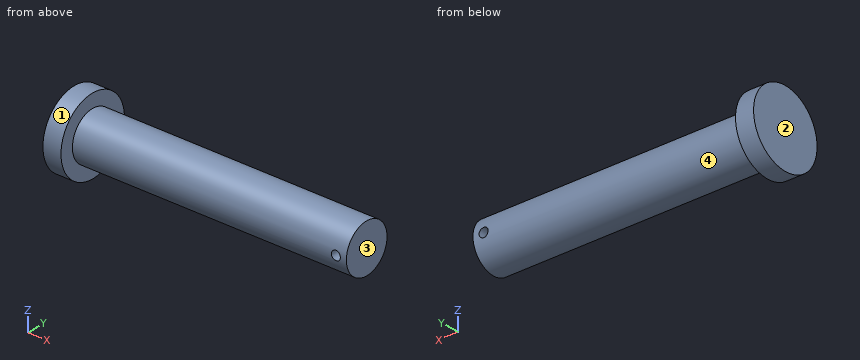
Autodesk Inventor part; units mm, degrees
ref_plane "Work Plane1" through (0, 16, 0) normal (0, 1, 0) x (-1, 0, 0)
ref_plane "YZ Plane" through (0, 0, 0) normal (1, 0, 0) x (0, 1, 0)
ref_plane "XY Plane" through (0, 0, 0) normal (0, 0, 1) x (1, 0, 0)
sketch "Sketch1" plane through (0, 0, 0) normal (1, 0, 0) x (0, 1, 0)
  line L0 (0, 35) -> (0, -35)
  line L1 (-35, 0) -> (35, 0)
  circle A0 centre (0, 0) radius 25
  dimension "d0" = 50
extrude "Extrusion1" add sketch "Sketch1" along normal blind 12
sketch "Sketch2" plane through (12, 0, 0) normal (1, 0, 0) x (0, 0, -1)
  circle A0 centre (0, 0) radius 16
  dimension "d3" = 32
extrude "Extrusion2" add sketch "Sketch2" along normal blind 182
ref_plane "Work Plane1" through (0, 16, 0) normal (0, 1, 0) x (-1, 0, 0)
sketch "Sketch3" plane through (0, 16, 0) normal (0, 1, 0) x (-1, 0, 0)
  circle A0 centre (-187, 0) radius 3
  point P0 (0, 0)
  dimension "d7" = 6
extrude "Extrusion3" cut sketch "Sketch3" against normal through all
properties part number "Pin" material "Stainless Steel"
Input: part model. Units: mm. Frame: model coordinates. Face numbers are marked on the shaded views. A direction names the side the tool comes from. Coordinates: 2 decimals unless noted, no trailing zeros. Order: outer loops, then holes, each group sorted by start corner. A loop starts at its lowest first (then second) coordinate and runs counter-clockwise, first axis right, second up. Notation, with made-up numbers: M 67.5,25.5 L 101.5,25.5 A15 ccw 101.5,31.5 Z; hole C 45.25,43 d11. An arc over 180 degrees is marked long. Write item = value, one per line. Start each with the question number.
(1) Line query: line 1 along X through (y, z) = (8, 0); line 2 along Z through (x, y) = (187, -0.5); line 3 along X through (y, z) = (17, 5). Output: solid intervals per line, ascending. Write a range as [from, to].
(2) First-contact query: P1, Ø1.5, axis at x = 154, z = -3, coming from the -Y side; P2, Ø12, axis at x = 171.5, z = -14.5, coming from the -Y side; P3, Ø10, axis at x = 121.5, z = 0, coming from the -Y side. Flat tips, straight axial feed; report the tip coordinate or a pass-through.
(3) Pull-direction query (Z, two-part tool) for the marked faces 1 and 2; classes: released by +Z, released by -Z, zero draft, split by the parting line, or undercut.
(4) Section C-C on x = 101. Output: boundary loops of the cut face in (y, z).
(5) Section A-A on z = 0. Output: boundary loops of the cut face in (x, y), and give its area (3 significant figures).
(6) Section B-B on y = 0. Output: boundary loops of the cut face in (x, z).
(7) Reachability of the marked faces 3 and 4 from +Z, -Z, +X, -X, +Y, -Y: full face, straight path, thin tool, end or side. Return the list, or none.
(8) Section D-D on z = 8.5. Output: boundary loops of the cut face in (x, y).
Result set:
q1.line_1 = [0, 184], [190, 194]
q1.line_2 = [-15.99, -3], [3, 15.99]
q1.line_3 = [0, 12]
q2.P1 = -15.84
q2.P2 = -13.56
q2.P3 = -16
q3.face_1 = split by the parting line
q3.face_2 = zero draft
q4.outline = C 0,0 d32
q5.outline = M 0,-25 L 12,-25 L 12,-16 L 184,-16 L 184,16 L 12,16 L 12,25 L 0,25 Z; M 190,-16 L 194,-16 L 194,16 L 190,16 Z
q5.area = 6,230 mm²
q6.outline = M 0,-25 L 12,-25 L 12,-16 L 194,-16 L 194,16 L 12,16 L 12,25 L 0,25 Z; hole C 187,0 d6
q7.face_3 = +Z, -Z, +X, +Y, -Y
q7.face_4 = +X
q8.outline = M 0,-23.51 L 12,-23.51 L 12,-13.56 L 194,-13.56 L 194,13.56 L 12,13.56 L 12,23.51 L 0,23.51 Z
